Work out the finished part from the listing and answer in its coordinate system (mm). Coordinates: 2 decimals unless noted, no trailing zeros. Order: outer loops, then holes, each group sorted by start corner. A loop starts at its lowest first (then second) coordinate and runs counter-clockwise, first axis right, second up. Notation, with made-up numbers: (70.5, -38.75) - (119.5, -38.75) arc R12 cw to (119.5, -29.75) - close; hole circle Ø9 at (49, -11). An arc over 180 degrees is marked (long way). Use CSV: the item, a comma, the result in double quotes. Start each with the question number.
from build123d import *

# Parameters (mm, degrees)
BOSS_EXTRUDE1_DEPTH = 10
FILLET2_R           = 5
FILLET3_R           = 5
FILLET4_R           = 5
FILLET5_R           = 5


with BuildPart() as part:
    # Sketch1 → Boss-Extrude1 (new body)
    with BuildSketch(Plane.XY):
        with BuildLine():
            Line((0, 10), (0, 5))
            Line((0, 5), (3, 5))
            ThreePointArc((3, 5), (4.5, 6.5), (6, 5))
            Line((6, 5), (136, 5))
            ThreePointArc((136, 5), (137.5, 6.5), (139, 5))
            Line((139, 5), (142, 5))
            Line((142, 5), (142, 10))
            Line((142, 10), (0, 10))
        make_face()
        with BuildLine():
            Line((3, 5), (0, 5))
            Line((0, 5), (0, 0))
            Line((0, 0), (142, 0))
            Line((142, 0), (142, 5))
            Line((142, 5), (139, 5))
            ThreePointArc((139, 5), (137.5, 3.5), (136, 5))
            Line((136, 5), (6, 5))
            ThreePointArc((6, 5), (4.5, 3.5), (3, 5))
        make_face()
    extrude(amount=BOSS_EXTRUDE1_DEPTH)

    # Fillet2
    fillet2_edges = [part.edges().sort_by_distance(p)[0] for p in [
        (0, 10, 5),
    ]]
    fillet(fillet2_edges, radius=FILLET2_R)

    # Fillet3
    fillet3_edges = [part.edges().sort_by_distance(p)[0] for p in [
        (0, 0, 5),
    ]]
    fillet(fillet3_edges, radius=FILLET3_R - 0.0001)  # a hair under: the kernel refuses the full size

    # Fillet4
    fillet4_edges = [part.edges().sort_by_distance(p)[0] for p in [
        (142, 10, 5),
    ]]
    fillet(fillet4_edges, radius=FILLET4_R)

    # Fillet5
    fillet5_edges = [part.edges().sort_by_distance(p)[0] for p in [
        (142, 0, 5),
    ]]
    fillet(fillet5_edges, radius=FILLET5_R - 0.0001)  # a hair under: the kernel refuses the full size


solid = part.part
1) The part is cut by section B-B on y = 8.5. Determine the outline of the cut face in (x, z), plus the area to 3 significant figures.
2) Straight lines are drawn through the part: line 1 (Y direction, x = 4.5, z = 5.5); line 2 (X direction, y = 4.5, z = 4.25); line 3 (X direction, y = 5.75, z = 9). For each, find the intervals that lie inside material, in ascending order. Write a range as [from, to].
3) Flat-ended cylindrical pins translate along their axes: P1, Ø3, axis at y = 9, z = 3, coming from the +X side; P2, Ø5, axis at y = 8, z = 8.5, coming from the -X side. Find the tip coordinate at first contact, or state that the pin passes through.
4) The part is cut by section A-A on z = 5.25. State how many separate pieces and enclosed holes the cut face has, plus the area to 3 significant figures.
5) For a pull along X with two mould halves and no side action, classify faces 1 (the face through (70, 0, 5)), 2 (the face through (136, 5, 5)), 3 (the face through (141, 2, 5)) as +X half, -X half, draft (parallel to the pull), parting line (faces both ways), or undercut.
Answer key:
1,outline,"(1.43, 0) - (140.57, 0) - (140.57, 10) - (1.43, 10) - close"
1,area,"1,390 mm^2"
2,line 1,"[0.03, 3.5], [6.5, 9.97]"
2,line 2,"[0.03, 3.09], [5.91, 136.09], [138.91, 141.97]"
2,line 3,"[0.06, 3.2], [5.8, 136.2], [138.8, 141.94]"
3,P1,"x = 141.33"
3,P2,"x = 0.03"
4,separate pieces,"1"
4,enclosed holes,"2"
4,area,"1,380 mm^2"
5,face 1,"draft"
5,face 2,"undercut"
5,face 3,"+X half"
